Autodesk Inventor part; units mm, degrees
ref_plane "YZ Plane" through (0, 0, 0) normal (1, 0, 0) x (0, 1, 0)
ref_plane "XZ Plane" through (0, 0, 0) normal (0, 1, 0) x (-1, 0, 0)
ref_plane "XY Plane" through (0, 0, 0) normal (0, 0, 1) x (1, 0, 0)
sketch "スケッチ1" plane through (0, 0, 0) normal (0, 0, 1) x (1, 0, 0)
  circle A0 centre (0, 0) radius 5
  circle A1 centre (0, 0) radius 3.75
  line L0 (-3.75, 3) -> (-2.75, 3)
  line L1 (-2.75, 3) -> (-2.75, -3)
  line L2 (-2.75, -3) -> (-3.75, -3)
  line L3 (-3.75, -3) -> (-3.75, 3)
  line L4 (3.75, -3) -> (2.75, -3)
  line L5 (2.75, -3) -> (2.75, 3)
  line L6 (2.75, 3) -> (3.75, 3)
  line L7 (3.75, 3) -> (3.75, -3)
  dimension "d0" = 10
  dimension "d1" = 7.5
  dimension "d2" = 5.5
  dimension "d3" = 1
  dimension "d4" = 1
  dimension "d5" = 6
  dimension "d6" = 6
  dimension "d7" = 3
  dimension "d8" = 2.75
  dimension "d17" = 3
extrude "押し出し1" add sketch "スケッチ1" against normal blind 3 contours A0 | A1 L5 | L7 L4 L5 A1 | A1 L5 L6 L7 | L1 A1 | A1 L3 L0 L1 | L1 L2 L3 A1
sketch "スケッチ2" plane through (0, 0, 0) normal (0, 0, 1) x (1, 0, 0)
  circle A0 centre (0, 0) radius 15
  circle A1 centre (0, 0) radius 4
  dimension "d11" = 30
  dimension "d14" = 8
extrude "押し出し3" add sketch "スケッチ2" against normal blind 1.5
properties part number "disc_put"
Source: CAD feature listing. Evaluate the final solid. Frame: model axes, mm. A direction names the side the tool comes from. Coordinates: 2 decimals unless noted, no trailing zeros. Loops run counter-clockwise (first coordinate to the right, second up) from the corner with the lowest first, then second, coordinate; pieces in that order, holes last. Notation, with made-up numbers: (80, 72.25) - (88, 72.25) arc R27 ccw to (88, 101.25) - close; hole circle Ø2 at (32.5, 32). An arc over 180 degrees is marked (long way). One line per item, written item: value. Start each with the question number.
1. Section D-D (z = -2.4). Return the cut outline in (x, y).
2. Section B-B (y = 0). Return the cut outline in (x, z).
3. Section C-C (z = -0.7). Return the cut outline in (x, y), and give its area (3 significant figures).
4. Contact query for flat-ended pins moving along their axis: P1, Ø1, axis at x = 9, z = -0.5, coming from the +Y side; P2, Ø1, axis at y = 3.5, z = -1, coming from the +X side; P3, Ø1.5, axis at y = 4, z = -1, coming from the +X side. Output: stop coordinate, or through.
5. Set-up query: faces 1 (the flat face through (3, 0, -3)), 2 (the flat face through (2.75, 0, -1)), 3 (the flat face through (-4, 4, -1.5)). Return all of +Z, -Z, +X, -X, +Y, -Y with unobstructed straight access to the full face (end or side cutting, diameter ignored); none if empty.
6. Mould query, pull axis X, two halves, no side actions, for faces 4 (the flat face through (3, 0, 0)), 5 (the cylindrical face through (-1.08, -4.88, -2.24)), 6 (the flat face through (-2.75, 0, -1)). Classes: pulls with the +X half, pulls with the -X half, needs draft (parallel to the pull), parting line crosses it, or undercut.
7. Section A-A (x = 0). Return the cut outline in (y, z), and give its area (3 significant figures).
8. Ray query, L1, parallel to Z at x = -9.5, y = -9.5; L2, parallel to Y at x = 2, z = -0.5; L3, parallel to X at y = -2, z = -2.6. Return the intervals inside material, ascending.
Verdict:
1. outline: circle Ø10 at (0, 0); hole (-2.75, -2.55) arc R3.75 ccw to (2.75, -2.55) - (2.75, 2.55) arc R3.75 ccw to (-2.75, 2.55) - close
2. outline: (-15, -1.5) - (-5, -1.5) - (-5, -3) - (-2.75, -3) - (-2.75, 0) - (-15, 0) - close; (2.75, -3) - (5, -3) - (5, -1.5) - (15, -1.5) - (15, 0) - (2.75, 0) - close
3. outline: circle Ø30 at (0, 0); hole (-2.75, -2.55) arc R3.75 ccw to (2.75, -2.55) - (2.75, 2.55) arc R3.75 ccw to (-2.75, 2.55) - close
3. area: 670 mm2
4. P1: stops at y = 12.36
4. P2: stops at x = 14.7
4. P3: stops at x = 14.64
5. face 1: -Z, +X, -X, +Y, -Y
5. face 2: +Z, -Z
5. face 3: -Z
6. face 4: needs draft
6. face 5: parting line crosses it
6. face 6: undercut
7. outline: (-15, -1.5) - (-5, -1.5) - (-5, -3) - (-3.75, -3) - (-3.75, 0) - (-15, 0) - close; (3.75, -3) - (5, -3) - (5, -1.5) - (15, -1.5) - (15, 0) - (3.75, 0) - close
7. area: 37.5 mm2
8. L1: z = -1.5 to 0
8. L2: y = -14.87 to -3.17, 3.17 to 14.87
8. L3: x = -4.58 to -2.75, 2.75 to 4.58
